The figure shows three views and two pictorial views of one solid part (mm, origin at its lowest corner). Answer the questions. A direction names the side the tool comes from. Round coordinates to 2 decimals unless told otherwise and drop trailing zeros. Order: outer loops, then holes, each group sorted by start corner. A loop starts at its lowest first (then second) coordinate and runs counter-clockwise, first axis right, second up. Notation, with made-up numbers: (73.25, 10) - (80.25, 10) arc R15 ccw to (80.25, 28) - close; hole circle Ø10 at (-31.75, 3). An arc over 180 degrees is marked (long way). Use CSV: the item, a comma, the result in double quotes.
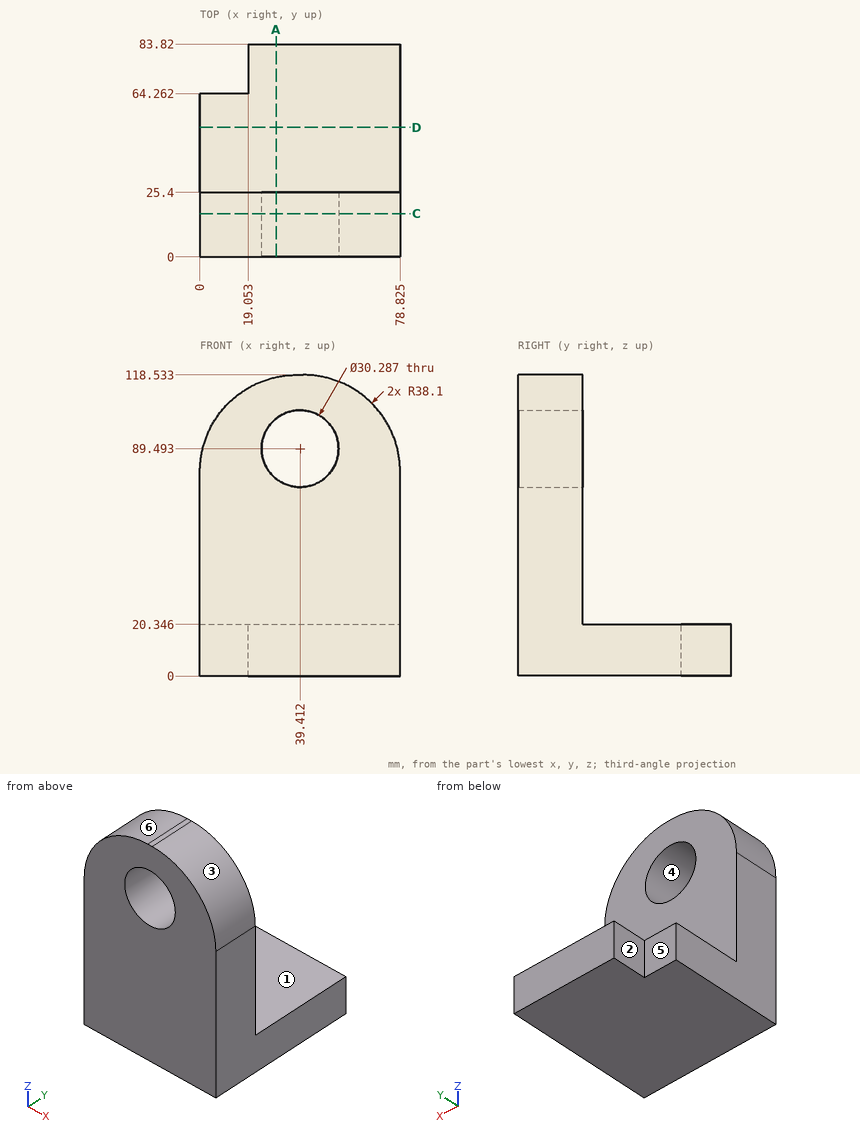
(1) Find section C-C (y = 17). Determine the outline of the cut face in (x, z) (1 decimal), and give its area (3 significant figures).
Findings below:
outline,"(0, 0) - (78.8, 0) - (78.8, 80.4) arc R38.1 ccw to (40.7, 118.5) - (38.1, 118.5) arc R38.1 ccw to (0, 80.4) - close; hole circle Ø30.3 at (39.4, 89.5)"
area,"8,000 mm²"
(2) Find section D-D (y = 51). Determine the outline of the cut face in (x, z) (1 decimal), and give its area (3 significant figures).
Findings below:
outline,"(0, 0) - (78.8, 0) - (78.8, 20.3) - (0, 20.3) - close"
area,"1,600 mm²"
(3) Find the intervals of material crossed by L1, parallel to Y at x = 15, z = 44; L2, parallel to Z at x = 15, y = 57 (1 decimal); L3, parallel to X at y = 21, z = 77 (1 decimal), in increasing order. Write a range as from..to.
Findings below:
L1,"y = 0..25.4"
L2,"z = 0..20.3"
L3,"x = 0..30.9, 48..78.8"
(4) For the marked faces 1, 2 and 3, determine the directions among +Z, -Z, +X, -X, +Y, -Y from which every point of the face is accessible in a straight line to the end or side of a thin tool.
Findings below:
face 1,"+Z, +X, -X, +Y"
face 2,"+Z, -Z, -X, +Y"
face 3,"+Z, +X, +Y, -Y"
(5) Each of these flat-tipped pins is pushed along its axis until it touches: pin 1 (1.5 mm diameter, centred on x = 47.5, z = 67, fed in from -Y); pin 2 (8 mm diameter, centred on x = 28.5, y = 30.5, fed in from +Z). Where does it stop, or does it pass through?
Findings below:
pin 1,"stops at y = 0"
pin 2,"stops at z = 20.35"
(6) Find section A-A (x = 30). Determine the outline of the cut face in (y, z) (1 decimal), and give its area (3 significant figures).
Findings below:
outline,"(0, 0) - (83.8, 0) - (83.8, 20.3) - (25.4, 20.3) - (25.4, 77.6) - (0, 77.6) - close; (0, 101.4) - (25.4, 101.4) - (25.4, 117.7) - (0, 117.7) - close"
area,"3,570 mm²"
(7) The mould has two halves that part along Z. Classify the marked faces 4, 5 and 6: released by +Z, released by -Z, zero draft, split by the parting line, or undercut.
Findings below:
face 4,"undercut"
face 5,"zero draft"
face 6,"released by +Z"
